Solid Edge part; units mm, degrees
sketch "Sketch1" plane through (0, 0, 0) normal (0, -1, 0) x (1, 0, 0)
  arc A0 (-27.5, 35) -> (-35, 27.5) centre (-27.5, 27.5) ccw
  line L0 (-35, 27.5) -> (-35, -27.5)
  arc A1 (-35, -27.5) -> (-27.5, -35) centre (-27.5, -27.5) ccw
  line L1 (-27.5, -35) -> (27.5, -35)
  arc A2 (27.5, -35) -> (35, -27.5) centre (27.5, -27.5) ccw
  line L2 (35, -27.5) -> (35, 27.5)
  arc A3 (35, 27.5) -> (27.5, 35) centre (27.5, 27.5) ccw
  line L3 (27.5, 35) -> (-27.5, 35)
  arc A4 (-27.5, 40) -> (-40, 27.5) centre (-27.5, 27.5) ccw
  line L4 (-40, 27.5) -> (-40, -27.5)
  arc A5 (-40, -27.5) -> (-27.5, -40) centre (-27.5, -27.5) ccw
  line L5 (-27.5, -40) -> (27.5, -40)
  arc A6 (27.5, -40) -> (40, -27.5) centre (27.5, -27.5) ccw
  line L6 (40, -27.5) -> (40, 27.5)
  arc A7 (40, 27.5) -> (27.5, 40) centre (27.5, 27.5) ccw
  line L7 (27.5, 40) -> (-27.5, 40)
extrude "Protrusion1" add sketch "Sketch1" against normal blind 47.625
Can you work these out from the model? Positions are in its coordinate system, mm. A direction names the side the tool comes from. Give positions to 0.01 mm unless a question says otherwise; leave off trailing zeros. Loops run counter-clockwise (first coordinate to the right, second up) from the corner with the lowest first, then second, coordinate; pieces in that order, holes last. Notation, with made-up numbers: (89, 16) -> (108, 16) arc R8 cw to (108, 30) -> close; hole circle Ø10 at (79, -4). An arc over 180 degrees is marked (long way). Return JSON: item names as keys, results as strings.
Q1. I want a section at C-C, the plane y = 18. List the corners of the cut face in (x, z) for me.
Checks:
{"outline": "(-40, -27.5) arc R12.5 ccw to (-27.5, -40) -> (27.5, -40) arc R12.5 ccw to (40, -27.5) -> (40, 27.5) arc R12.5 ccw to (27.5, 40) -> (-27.5, 40) arc R12.5 ccw to (-40, 27.5) -> close; hole (-35, -27.5) arc R7.5 ccw to (-27.5, -35) -> (27.5, -35) arc R7.5 ccw to (35, -27.5) -> (35, 27.5) arc R7.5 ccw to (27.5, 35) -> (-27.5, 35) arc R7.5 ccw to (-35, 27.5) -> close"}
Q2. On a 3-axis mill with a long thin cutter (end or side, diameter ignored), from which of +Z, -Z, +X, -X, +Y, -Y can I reach the whole of each face in a straight line? I mean faces 4 (the face through (-32.861, 23.479, -32.745)), 5 (the face through (0, 47.625, 36)). Say none if no direction works.
Checks:
{"face 4": "+Y, -Y", "face 5": "+Z, -Z, +X, -X, +Y"}
Q3. I want a section at B-B, the plane x = -5.5. List the corners of the cut face in (y, z) for me (3 decimals), then the cut area to 3 significant figures.
Checks:
{"outline": "(0, -40) -> (47.625, -40) -> (47.625, -35) -> (0, -35) -> close; (0, 35) -> (47.625, 35) -> (47.625, 40) -> (0, 40) -> close", "area": "476 mm2"}
Q4. For pin 1 Ø6 at (y, z) = (16, -32) entering from +X, with a flat end and sliding along its axis, tell me the tip position at first contact or that it passes through.
Checks:
{"pin 1": "stops at x = 39.91"}
Q5. I want a section at A-A, the plane z = 5. List the corners of the cut face in (x, y) for me (3 decimals).
Checks:
{"outline": "(-40, 0) -> (-35, 0) -> (-35, 47.625) -> (-40, 47.625) -> close; (35, 0) -> (40, 0) -> (40, 47.625) -> (35, 47.625) -> close"}
Q6. I need wall thicknesses on probe 1 along X at (y, z) = (14.5, 28); probe 2 along Z at (x, y) = (-16, 14.5); probe 3 along Z at (x, y) = (29, 32.5). Which ranges of each line are inside material? Lowest first, please.
Checks:
{"probe 1": "x = -39.99 to -34.98, 34.98 to 39.99", "probe 2": "z = -40 to -35, 35 to 40", "probe 3": "z = -39.91 to -34.85, 34.85 to 39.91"}
Q7. We'd pull the mould along X, two halves only. Please class faces 1 (the face through (0, 0, 36)), 2 (the face through (32.745, 23.479, -32.861)), 3 (the face through (-40, 23, 0)): released by +X, released by -X, zero draft, split by the parting line, or undercut.
Checks:
{"face 1": "zero draft", "face 2": "undercut", "face 3": "released by -X"}
